from build123d import *

# Parameters (mm, degrees)
F0_W     = 92
F0_H     = 23.8
F1_DEPTH = 0.42
F2_W     = 70.4
F2_H     = 23
F2_W_2   = 68
F2_H_2   = 20.2
F3_DEPTH = 5
F4_W     = 68
F4_H     = 20.2
F5_DEPTH = 25


with BuildPart() as f1:
    # F0 (on Top) → F1 (new body)
    with BuildSketch(Plane.XY):
        Rectangle(F0_W, F0_H)
    extrude(amount=F1_DEPTH)

    # F2 (on face) → F3 (join)
    with BuildSketch(Plane.XY.offset(0.42)):
        Rectangle(F2_W, F2_H)
        Rectangle(F2_W_2, F2_H_2, mode=Mode.SUBTRACT)
    extrude(amount=F3_DEPTH)

    # F4 (on face) → F5 (cut)
    with BuildSketch(Plane.XY.offset(0.42)):
        Rectangle(F4_W, F4_H)
    extrude(amount=-F5_DEPTH, mode=Mode.SUBTRACT)


solid = f1.part
Work out the finished part from the listing and answer in its coordinate system (mm). A direction names the side the tool comes from. Round coordinates to 2 decimals unless told otherwise and drop trailing zeros. Write each loop counter-clockwise with the first axis right and the second up, starting at its lowest first coordinate (ties: lowest second). Pieces come first, ordered by that corner, then holes.
1) The mould has two halves that part along X. Classify faces 4 (the flat face through (-8, 10.3, 5.42)), 5 (the flat face through (34, 0, 3)), 6 (the flat face through (35.2, 0, 3)): pulls with the +X half, pulls with the -X half, needs draft (parallel to the pull), parting line crosses it, or undercut.
2) A tool of negligible diameter and unlimited length cuts with its end or side. For faces 1 (the flat face through (0, 11.5, 3)), 2 (the flat face through (-35.2, 0, 3)), 3 (the flat face through (0, -10.1, 3)), from which of +Z, -Z, +X, -X, +Y, -Y can it reach the whole face along a straight path? Write none if from no direction.
3) A cutting plane is placed at C-C (z = 1.45). Give the vertices of the cut face in (x, y).
4) A cutting plane is placed at A-A (y = 9). Give the vertices of the cut face in (x, z).
5) A cutting plane is placed at D-D (x = -39). Give the vertices of the cut face in (y, z), plus the area to 4 significant figures.
6) A cutting plane is placed at B-B (x = 3). Give the vertices of the cut face in (y, z), plus the area to 3 significant figures.
7) Straight lines are drawn through the part: line 1 (Y direction, x = -17.5, z = 0.85); line 2 (X direction, y = 7.5, z = 2.2); line 3 (X direction, y = -7, z = 0.3). For each, find the intervals that lie inside material, in ascending order.
8) Given pin 1 Ø7 at (x, y) = (-1.5, -5) entering from +Z; pin 2 Ø2.5 at (x, z) = (9.5, 2) entering from +Y; pin 3 Ø2 at (y, z) = (8, 4.5) entering from -X, each flat-ended and moving along its own axis, determine where each tip first touches the part or whether it passes through.
Completed:
1. face 4: needs draft
1. face 5: undercut
1. face 6: pulls with the +X half
2. face 1: +Z, +X, -X, +Y
2. face 2: +Z, -X, +Y, -Y
2. face 3: +Z, -Z
3. outline: (-35.2, -11.5) - (35.2, -11.5) - (35.2, 11.5) - (-35.2, 11.5) - close; hole (-34, -10.1) - (34, -10.1) - (34, 10.1) - (-34, 10.1) - close
4. outline: (-46, 0) - (-34, 0) - (-34, 5.42) - (-35.2, 5.42) - (-35.2, 0.42) - (-46, 0.42) - close; (34, 0) - (46, 0) - (46, 0.42) - (35.2, 0.42) - (35.2, 5.42) - (34, 5.42) - close
5. outline: (-11.9, 0) - (11.9, 0) - (11.9, 0.42) - (-11.9, 0.42) - close
5. area: 10.00 mm2
6. outline: (-11.9, 0) - (-10.1, 0) - (-10.1, 5.42) - (-11.5, 5.42) - (-11.5, 0.42) - (-11.9, 0.42) - close; (10.1, 0) - (11.9, 0) - (11.9, 0.42) - (11.5, 0.42) - (11.5, 5.42) - (10.1, 5.42) - close
6. area: 15.5 mm2
7. line 1: y = -11.5 to -10.1, 10.1 to 11.5
7. line 2: x = -35.2 to -34, 34 to 35.2
7. line 3: x = -46 to -34, 34 to 46
8. pin 1: passes through
8. pin 2: stops at y = 11.5
8. pin 3: stops at x = -35.2
